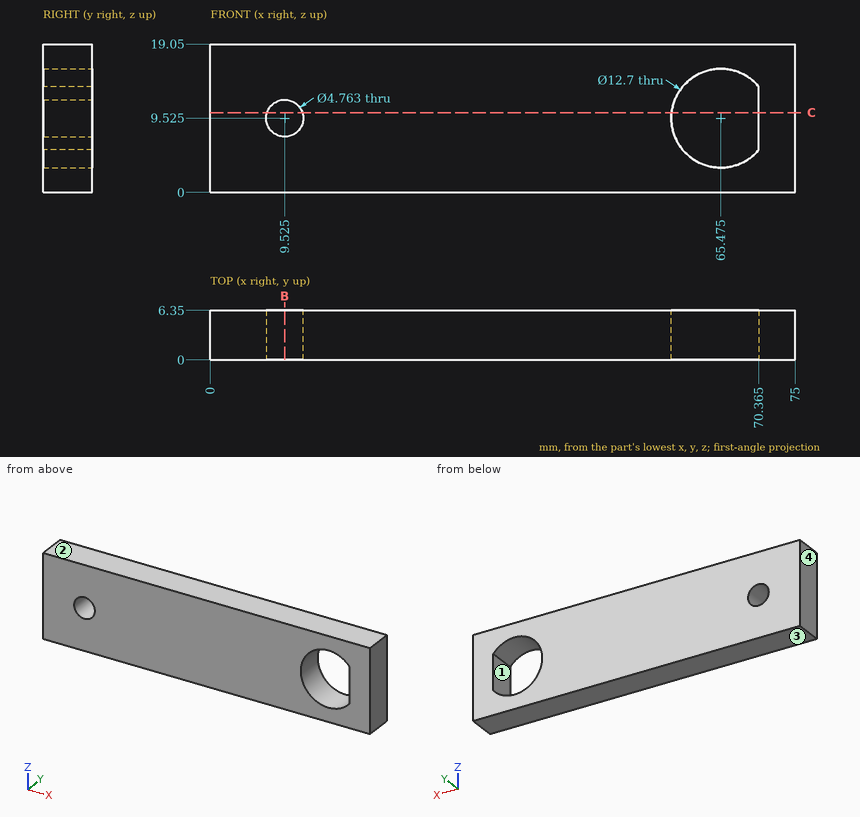
Answer from the drawing. Dimensions are ordinates in mm from the lowest x, y and z of the part. Coordinates: 2 decimals unless noted, no trailing zeros. Order: outer loops, then holes, each group sorted by start corner. A loop starts at its lowest first (then second) coordinate and runs counter-clockwise, first axis right, second up. Notation, with made-up numbers: (-17, 68.5) -> (2, 68.5) arc R22 cw to (2, 87.5) -> close; hole circle Ø9 at (59, 38). An arc over 180 degrees is marked (long way). Answer as a JSON object with one key per item and string values.
1) A cutting plane is placed at C-C, the plane z = 10.25. State how many separate pieces and enclosed holes the cut face has, plus the area to 3 significant figures.
Model answer:
{"separate pieces": "3", "enclosed holes": "0", "area": "376 mm²"}
2) This flat-tipped pin is pushed along its axis until it touches: pin 1 (10 mm diameter, centred on x = 65.475, z = 9.525, fed in from -Y). Where does it stop, or does it pass through?
Model answer:
{"pin 1": "stops at y = 0"}
3) The mould has two halves that part along Z. Classify the marked faces 1, 2, 3 and 4: released by +Z, released by -Z, zero draft, split by the parting line, or undercut.
Model answer:
{"face 1": "undercut", "face 2": "released by +Z", "face 3": "released by -Z", "face 4": "zero draft"}
4) A cutting plane is placed at B-B, the plane x = 9.5. Determine the outline of the cut face in (y, z).
Model answer:
{"outline": "(0, 0) -> (6.35, 0) -> (6.35, 7.14) -> (0, 7.14) -> close; (0, 11.91) -> (6.35, 11.91) -> (6.35, 19.05) -> (0, 19.05) -> close"}
5) Consider line 1 along X through (y, z) = (2, 8.5) (1 decimal); line 2 along X through (y, z) = (2.5, 4.5) (1 decimal); line 3 along X through (y, z) = (1, 5). Determine where each line is inside the solid, lowest interval first. Write a range as from..to.
Model answer:
{"line 1": "x = 0..7.4, 11.7..59.2, 70.4..75", "line 2": "x = 0..61.6, 69.4..75", "line 3": "x = 0..61.02, 69.93..75"}
